Design review of the part built by this model. Coordinates are the model's own, in mm. A direction names the side the tool comes from. Give positions to 0.01 mm unless a question says otherwise; leave off trailing zeros. Write each loop counter-clockwise with the first axis right and the second up, starting at its lowest first coordinate (ties: lowest second). Pieces come first, ordered by that corner, then holes. Notation, with made-up numbers: (-10, -10.5) -> (1, -10.5) arc R29 cw to (1, 28.5) -> close; hole circle Ø8 at (-26.5, 35.5). An arc over 180 degrees is marked (long way). Write each question's results on one line, items separated by ' | '. Start each with the question number.
(1) For faces 4 (the face through (6.304, -6.424, 0.986)), 5 (the face through (-3, 3, 0)), 6 (the face through (-2.17, -9.76, 5.94)), list the 3-axis set-ups (+Z, -Z, +X, -X, +Y, -Y) from which the entire face can be reached by the end or side of a thin tool; tool diameter is ignored.
(2) Take a section at C-C (y = -4.75). State the section outline as (x, z) points, plus the area to 3 significant figures.
(3) Take a section at A-A (y = 0). State the section outline as (x, z) points.
(4) To check wall thickness, follow probe 1 along Y at (x, z) = (0, 4.75); probe 2 along Y at (x, z) = (-4, 1); probe 3 along Y at (x, z) = (0, 0.6). State the ranges of each line that lie inside material, in increasing order.
(5) Clearance check with flat-ended pins moving along their axes: pin 1 (1 mm diameter, centred on y = -8, z = 1.5, fed in from -X); pin 2 (1 mm diameter, centred on x = -8, z = 1, fed in from +Y); pin 3 (2 mm diameter, centred on x = 8, z = 3, fed in from -Y); pin 4 (5 mm diameter, centred on x = -2.5, y = 1, fed in from -Z). State where each tip first meets the part, or that it passes through.
(6) Take a section at D-D (z = 1.5). State the section outline as (x, y) points, plus the area to 3 significant figures.
(7) Mouldability with a two-part tool opening along X and no side actions: class faces 1 (the face through (2, -10, 10)), 2 (the face through (-1, -7, 1)), 3 (the face through (-2.38, -10.74, 4.93)) as released by +X, released by -X, zero draft, split by the parting line, or undercut.
from build123d import *

# Parameters (mm, degrees)
ESBO_O1_R                = 10
ESBO_O1_R_2              = 3.65
RESSALTO_EXTRUS_O1_DEPTH = 2
ESBO_O2_R                = 11
ESBO_O2_R_2              = 10
RESSALTO_EXTRUS_O2_DEPTH = 10
CORTE_EXTRUS_O1_DEPTH    = 10


with BuildPart() as part:
    # Esboço1 → Ressalto-extrusão1 (new body)
    with BuildSketch(Plane.XY):
        Circle(ESBO_O1_R)
        Circle(ESBO_O1_R_2, mode=Mode.SUBTRACT)
    extrude(amount=RESSALTO_EXTRUS_O1_DEPTH)

    # Esboço2 → Ressalto-extrusão2 (add)
    with BuildSketch(Plane.XY):
        Circle(ESBO_O2_R)
        Circle(ESBO_O2_R_2, mode=Mode.SUBTRACT)
    extrude(amount=RESSALTO_EXTRUS_O2_DEPTH)

    # Esboço3 → Corte-extrusão1 (cut)
    with BuildSketch(Plane(origin=(0, 0, 0), x_dir=(-1, 0, 0), z_dir=(0, 0, -1))):
        with BuildLine():
            Line((-8.94427191, -1), (-6, -1))
            Line((-6, -1), (-5.916079783, -1))
            ThreePointArc((-5.916079783, -1), (-4.242640687, -4.242640687), (-1, -5.916079783))
            Line((-1, -5.916079783), (-1, -6))
            Line((-1, -6), (-1, -8.94427191))
            ThreePointArc((-1, -8.94427191), (-6.363961031, -6.363961031), (-8.94427191, -1))
        make_face()
        with BuildLine():
            Line((-8.94427191, 1), (-6, 1))
            Line((-6, 1), (-5.916079783, 1))
            ThreePointArc((-5.916079783, 1), (-4.242640687, 4.242640687), (-1, 5.916079783))
            Line((-1, 5.916079783), (-1, 6))
            Line((-1, 6), (-1, 8.94427191))
            ThreePointArc((-1, 8.94427191), (-6.363961031, 6.363961031), (-8.94427191, 1))
        make_face()
        with BuildLine():
            Line((1, 6), (1, 8.94427191))
            ThreePointArc((1, 8.94427191), (6.363961031, 6.363961031), (8.94427191, 1))
            Line((8.94427191, 1), (6, 1))
            Line((6, 1), (5.916079783, 1))
            ThreePointArc((5.916079783, 1), (4.242640687, 4.242640687), (1, 5.916079783))
            Line((1, 5.916079783), (1, 6))
        make_face()
        with BuildLine():
            Line((6, -1), (8.94427191, -1))
            ThreePointArc((8.94427191, -1), (6.363961031, -6.363961031), (1, -8.94427191))
            Line((1, -8.94427191), (1, -6))
            Line((1, -6), (1, -5.916079783))
            ThreePointArc((1, -5.916079783), (4.242640687, -4.242640687), (5.916079783, -1))
            Line((5.916079783, -1), (6, -1))
        make_face()
    extrude(amount=-CORTE_EXTRUS_O1_DEPTH, mode=Mode.SUBTRACT)


solid = part.part
Report:
1) face 4: +Z, -Z | face 5: -Z, +X, -X, +Y, -Y | face 6: +Z
2) outline: (-9.92, 0) -> (-7.64, 0) -> (-7.64, 2) -> (-8.8, 2) -> (-8.8, 10) -> (-9.92, 10) -> close; (-3.67, 0) -> (3.67, 0) -> (3.67, 2) -> (-3.67, 2) -> close; (7.64, 0) -> (9.92, 0) -> (9.92, 10) -> (8.8, 10) -> (8.8, 2) -> (7.64, 2) -> close | area: 41.7 mm2
3) outline: (-11, 0) -> (-3.65, 0) -> (-3.65, 2) -> (-10, 2) -> (-10, 10) -> (-11, 10) -> close; (3.65, 0) -> (11, 0) -> (11, 10) -> (10, 10) -> (10, 2) -> (3.65, 2) -> close
4) probe 1: -11 to -10, 10 to 11 | probe 2: -10.25 to -8.06, -4.47 to 4.47, 8.06 to 10.25 | probe 3: -11 to -3.65, 3.65 to 11
5) pin 1: x = -8.05 | pin 2: y = 8.05 | pin 3: y = -8.49 | pin 4: z = 0
6) outline: circle Ø22 at (0, 0); hole (-8.94, -1) arc R9 ccw to (-1, -8.94) -> (-1, -5.92) arc R6 cw to (-5.92, -1) -> close; hole (-8.94, 1) -> (-5.92, 1) arc R6 cw to (-1, 5.92) -> (-1, 8.94) arc R9 ccw to start; hole circle Ø7.3 at (0, 0); hole (1, -8.94) arc R9 ccw to (8.94, -1) -> (5.92, -1) arc R6 cw to (1, -5.92) -> close; hole (1, 5.92) arc R6 cw to (5.92, 1) -> (8.94, 1) arc R9 ccw to (1, 8.94) -> close | area: 221 mm2
7) face 1: zero draft | face 2: undercut | face 3: split by the parting line
